For this review, take the finished solid that the model builds, in its own axes (mm). A direction names the side the tool comes from. Coordinates: 2 decimals unless noted, no trailing zeros. Write each loop counter-clockwise with the first axis right and the second up, starting at its lowest first coordinate (ties: lowest second). Pieces come first, ordered by that corner, then holes.
```python
from build123d import *

# Parameters (mm, degrees)
BOSS_EXTRUDE1_DEPTH = 2.5
BOSS_EXTRUDE2_DEPTH = 85


with BuildPart() as part:
    # Sketch1 → Boss-Extrude1 (new, symmetric)
    with BuildSketch(Plane(origin=(0, 0, 0), x_dir=(1, 0, 0), z_dir=(0, 1, 0))):
        with BuildLine():
            Line((-46.169490158, -34.493062002), (-69.80030965, 22.556782905))
            ThreePointArc((-69.80030965, 22.556782905), (-1.110079213, 35.825157058), (67.580151223, 22.556782905))
            Line((67.580151223, 22.556782905), (43.949331732, -34.493062002))
            ThreePointArc((43.949331732, -34.493062002), (-1.110079213, -27.613322498), (-46.169490158, -34.493062002))
        make_face()
    boss_extrude1 = extrude(amount=BOSS_EXTRUDE1_DEPTH, both=True)

    # Sketch2 → Boss-Extrude2 (add)
    with BuildSketch(Plane(origin=(0, 2.5, 0), x_dir=(1, 0, 0), z_dir=(0, 1, 0))):
        with BuildLine():
            Line((-29.32170103, 3.22655488), (-28.133506793, 0.358000238))
            ThreePointArc((-28.133506793, 0.358000238), (-1.110079213, 2.386677502), (25.913348366, 0.358000238))
            Line((25.913348366, 0.358000238), (27.101542603, 3.22655488))
            ThreePointArc((27.101542603, 3.22655488), (-1.110079213, 5.825157058), (-29.32170103, 3.22655488))
        make_face()
    extrude(amount=BOSS_EXTRUDE2_DEPTH)

    # Mirror1: Boss-Extrude1 across plane
    add(boss_extrude1.mirror(Plane.ZX.offset(45)))


solid = part.part
```
Q1. Add section A-A (z = -19.5). State the section outline as (x, y) points, then the cut area to 3 significant figures.
Ans:
outline: (-68.53, -2.5) - (66.31, -2.5) - (66.31, 2.5) - (-68.53, 2.5) - close; (-68.53, 87.5) - (66.31, 87.5) - (66.31, 92.5) - (-68.53, 92.5) - close
area: 1,350 mm2
Q2. For probe 1 along Y at (x, z) = (42, 21.5); probe 2 along Z at (x, y) = (-3, 84.5); probe 3 along Z at (x, y) = (-13, 27), list the stretches that pass through material, from the lowest coordinate up.
Ans:
probe 1: y = -2.5 to 2.5, 87.5 to 92.5
probe 2: z = -5.81 to -2.38
probe 3: z = -5.37 to -2
Q3. Add section B-B (x = -43.5). State the section outline as (y, z) points, then the cut area to 3 significant figures.
Ans:
outline: (-2.5, -30.89) - (2.5, -30.89) - (2.5, 33.69) - (-2.5, 33.69) - close; (87.5, -30.89) - (92.5, -30.89) - (92.5, 33.69) - (87.5, 33.69) - close
area: 646 mm2
Q4. Tool access review of faces 1 (the cylindrical face through (-0.713, 44.405, -5.825)), 2 (the flat face through (0, 92.5, -1)), 3 (the flat face through (-28.736, 44.405, -1.812)), 4 (the cylindrical face through (-0.469, 89.965, 27.615)), 5 (the flat face through (26.5, 44.4, -1.77)): name each direction out of +Z, -Z, +X, -X, +Y, -Y from which nothing blocks a thin tool from reaching the whole face with its end or side.
Ans:
face 1: -Z
face 2: +Z, -Z, +X, -X, +Y
face 3: +Z, -X
face 4: +Z, +Y, -Y
face 5: +Z, +X
Q5. Draft analysis for pull direction X (two halves, no side actions). For faces 6 (the cylindrical face through (-1.49, 44.405, -2.386)), 7 (the cylindrical face through (-2.095, 89.965, -35.823)), 8 (the flat face through (-57.82, 89.96, 6.37)), state which applies: +X half, -X half, draft (parallel to the pull), parting line (faces both ways), or undercut.
Ans:
face 6: undercut
face 7: parting line
face 8: -X half
Q6. Add section D-D (y = 38). State the section outline as (x, z) points, then the cut area to 3 significant figures.
Ans:
outline: (-29.32, -3.23) arc R154.44 ccw to (27.1, -3.23) - (25.91, -0.36) arc R181 cw to (-28.13, -0.36) - close
area: 183 mm2
Q7. Add section C-C (x = 6). State the section outline as (y, z) points, then the cut area to 3 significant figures.
Ans:
outline: (-2.5, -35.69) - (2.5, -35.69) - (2.5, -5.66) - (87.5, -5.66) - (87.5, -35.69) - (92.5, -35.69) - (92.5, 27.78) - (87.5, 27.78) - (87.5, -2.25) - (2.5, -2.25) - (2.5, 27.78) - (-2.5, 27.78) - close
area: 925 mm2
